The model under review builds one solid part; all positions refer to its coordinate system, in mm. A direction names the side the tool comes from. Coordinates: 2 decimals unless noted, no trailing zeros. Loops run counter-clockwise (first coordinate to the right, second up) from the corner with the lowest first, then second, coordinate; pieces in that order, holes last. Notation, with made-up numbers: M 63.5,2 L 87.5,2 A12 cw 87.5,18 Z; hole C 14,-27.75 d11. An arc over 180 degrees is marked long. Use CSV: the item, a comma, the result in double quotes. Start each with the question number.
1. Tool access review of faces 5 (the cylindrical face through (-3.62, 46.98, 2.08)), 6 (the flat face through (-23.575, 38, 2)), 7 (the cylindrical face through (-44.201, 38.467, 2.079)): name each direction out of +Z, -Z, +X, -X, +Y, -Y from which nothing blocks a thin tool from reaching the whole face with its end or side.
2. For L1, parallel to X at y = 29, z = 3 (3 decimals); L2, parallel to Y at x = -59, z = 3.05; L3, parallel to X at y = 16, z = 3.4, list the stretches that pass through material, from the lowest coordinate up.
3. Add section B-B, the plane y = 18.5. Write out the cut boundary in (x, z), then the cut area to 3 significant figures.
4. Add section C-C, the plane x = -123.5. Write out the cut boundary in (y, z).
5. Add section A-A, the plane x = -67. Write out the cut boundary in (y, z), then the cut area to 3 significant figures.
6. Clearance check with flat-ended pins moving along their axes: P1, Ø1.3, axis at y = 39.5, z = 2.5, coming from the +X side; P2, Ø1.3, axis at y = 43, z = 1.5, coming from the -X side. State where each tip first meets the part, or that it passes through.
7. Draft analysis for pull direction Y (two halves, no side actions). For faces 1 (the cylindrical face through (-108.199, 9.793, 2.079)), 2 (the flat face through (-128.825, 38, 2)), 3 (the flat face through (-76, 7.62, 2)), 4 (the cylindrical face through (-148.78, 3.82, 2.08)), state which applies: +Y half, -Y half, draft (parallel to the pull), parting line (faces both ways), or undercut.
from build123d import *

# Parameters (mm, degrees)
F1_DEPTH = 4.2164


with BuildPart() as f1:
    # F0 (on Top) → F1 (new body)
    with BuildSketch(Plane.XY):
        with BuildLine():
            Line((-128.825, 50.8), (-139.7, 50.8))
            ThreePointArc((-139.7, 50.8), (-148.680256, 47.080256), (-152.4, 38.1))
            Line((-152.4, 38.1), (-152.4, 12.7))
            ThreePointArc((-152.4, 12.7), (-148.680256, 3.719744), (-139.7, 0))
            Line((-139.7, 0), (-12.7, 0))
            ThreePointArc((-12.7, 0), (-3.719744, 3.719744), (0, 12.7))
            Line((0, 12.7), (0, 38.1))
            ThreePointArc((0, 38.1), (-3.719744, 47.080256), (-12.7, 50.8))
            Line((-12.7, 50.8), (-23.575, 50.8))
            Line((-23.575, 50.8), (-23.575, 25.4))
            ThreePointArc((-23.575, 25.4), (-28.575, 20.4), (-33.575, 25.4))
            Line((-33.575, 25.4), (-33.575, 50.8))
            Line((-33.575, 50.8), (-118.825, 50.8))
            Line((-118.825, 50.8), (-118.825, 25.4))
            ThreePointArc((-118.825, 25.4), (-123.825, 20.4), (-128.825, 25.4))
            Line((-128.825, 25.4), (-128.825, 50.8))
        make_face()
        with BuildLine():
            ThreePointArc((-110.49, 33.02), (-108.258154, 38.408154), (-102.87, 40.64))
            Line((-102.87, 40.64), (-49.53, 40.64))
            ThreePointArc((-49.53, 40.64), (-44.141846, 38.408154), (-41.91, 33.02))
            Line((-41.91, 33.02), (-41.91, 15.24))
            ThreePointArc((-41.91, 15.24), (-44.141846, 9.851846), (-49.53, 7.62))
            Line((-49.53, 7.62), (-102.87, 7.62))
            ThreePointArc((-102.87, 7.62), (-108.258154, 9.851846), (-110.49, 15.24))
            Line((-110.49, 15.24), (-110.49, 33.02))
        make_face(mode=Mode.SUBTRACT)
    extrude(amount=F1_DEPTH)


solid = f1.part
Computed:
1,face 5,"+Z, -Z, +X, +Y"
1,face 6,"+Z, -Z, +Y"
1,face 7,"+Z, -Z"
2,L1,"x = -152.4 to -128.825, -118.825 to -110.49, -41.91 to -33.575, -23.575 to 0"
2,L2,"y = 0 to 7.62, 40.64 to 50.8"
2,L3,"x = -152.4 to -110.49, -41.91 to 0"
3,outline,"M -152.4,0 L -110.49,0 L -110.49,4.22 L -152.4,4.22 Z; M -41.91,0 L 0,0 L 0,4.22 L -41.91,4.22 Z"
3,area,"353 mm^2"
4,outline,"M 0,0 L 20.41,0 L 20.41,4.22 L 0,4.22 Z"
5,outline,"M 0,0 L 7.62,0 L 7.62,4.22 L 0,4.22 Z; M 40.64,0 L 50.8,0 L 50.8,4.22 L 40.64,4.22 Z"
5,area,"75.0 mm^2"
6,P1,"stops at x = -0.02"
6,P2,"stops at x = -151.67"
7,face 1,"undercut"
7,face 2,"draft"
7,face 3,"undercut"
7,face 4,"-Y half"
